Answer from the drawing. Dimensions are ordinates in mm from the lowest x, y and z of the part. A direction names the side the tool comes from. Give positions to 0.01 mm unless a question says otherwise; leave off trailing zeros. Loops run counter-clockwise (first coordinate to the right, second up) from the corner with the lowest first, then second, coordinate; pieces in that order, holes last. Notation, with made-up numbers: (9, 51.5) -> (34, 51.5) arc R22 ccw to (34, 72.5) -> close; hole circle Ø3 at (23, 45). An arc over 180 degrees is marked (long way). Return JSON: item names as keys, results as strings. Group by question number.
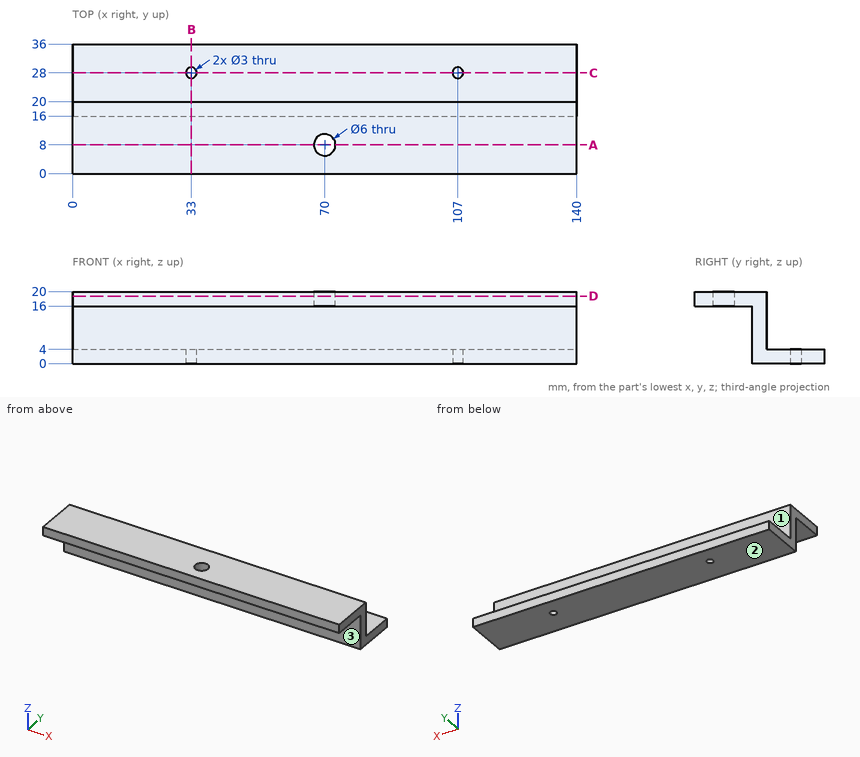
1. Section D-D on z = 18.75 is taken. Determine the outline of the cut face in (x, y), then the cut area to 3 significant figures.
2. Section B-B on x = 33 is taken. Determine the outline of the cut face in (y, z).
3. Section C-C on y = 28 is taken. Determine the outline of the cut face in (x, z).
4. Straight lines are drawn through the part: line 1 (Y direction, x = 70, z = 17.25); line 2 (Z direction, x = 110.5, y = 10.5); line 3 (Z direction, x = 92, y = 21). For each, find the intervals that lie inside material, in ascending order. Write a range as from..to.
5. Which of the six approach directions +Z, -Z, +X, -X, +Y, -Y give full straight-line access (tool end or side, diameter ignored) to the marked faces 1, 2 and 3?
6. Flat-ended cylindrical pins translate along their axes: pin 1 Ø4 at (x, y) = (21.5, 21) entering from +Z; pin 2 Ø3 at (x, z) = (46.5, 14) entering from -Y; pin 3 Ø8 at (x, y) = (22.5, 24.5) entering from +Z; pin 4 Ø13 at (x, y) = (72.5, 7.5) entering from -Z. Find the tip coordinate at first contact, or state that the pin passes through.
7. Section A-A on y = 8 is taken. Determine the outline of the cut face in (x, z), then the cut area to 3 significant figures.
Completed:
{
 "1": {"outline": "(0, 0) -> (140, 0) -> (140, 20) -> (0, 20) -> close; hole circle Ø6 at (70, 8)", "area": "2,770 mm²"},
 "2": {"outline": "(0, 16) -> (16, 16) -> (16, 0) -> (26.5, 0) -> (26.5, 4) -> (20, 4) -> (20, 20) -> (0, 20) -> close; (29.5, 0) -> (36, 0) -> (36, 4) -> (29.5, 4) -> close"},
 "3": {"outline": "(0, 0) -> (31.5, 0) -> (31.5, 4) -> (0, 4) -> close; (34.5, 0) -> (105.5, 0) -> (105.5, 4) -> (34.5, 4) -> close; (108.5, 0) -> (140, 0) -> (140, 4) -> (108.5, 4) -> close"},
 "4": {"line 1": "y = 0..5, 11..20", "line 2": "z = 16..20", "line 3": "z = 0..4"},
 "5": {"face 1": "+Z, +X, -X, +Y", "face 2": "-Z, +X, -X, +Y, -Y", "face 3": "-Z, +X, -X, -Y"},
 "6": {"pin 1": "stops at z = 20", "pin 2": "stops at y = 16", "pin 3": "stops at z = 4", "pin 4": "stops at z = 16"},
 "7": {"outline": "(0, 16) -> (67, 16) -> (67, 20) -> (0, 20) -> close; (73, 16) -> (140, 16) -> (140, 20) -> (73, 20) -> close", "area": "536 mm²"}
}
